Work out the finished part from the listing and answer in its coordinate system (mm). Face numbers are marked on the shaded views. A direction names the side the tool comes from. Give positions to 0.01 mm unless a question says otherwise; leave off trailing zeros. Loops run counter-clockwise (first coordinate to the right, second up) from the corner with the lowest first, then second, coordinate; pieces in that order, holes last. Notation, with made-up numbers: (-36.5, 73) -> (-3.5, 73) arc R17 cw to (-3.5, 96) -> close; hole circle Ø8 at (0.25, 19.5). An arc over 180 degrees is marked (long way). Answer as CSV lines item,"result". Start each with the question number.
1. Flat-ended cylindrical pins translate along their axes: pin 1 Ø0.6 at (y, z) = (1.5, 1) entering from -X; pin 2 Ø1.8 at (x, y) = (13, 2.5) entering from -Z; pin 3 Ø2 at (y, z) = (2, 6.5) entering from -X. Find the tip coordinate at first contact, or state that the pin passes through.
2. Find section A-A, the plane x = 0. Give the vertices of the cut face in (y, z).
3. Find section C-C, the plane z = 5.5. Give the vertices of the cut face in (x, y).
4. A tool of negligible diameter and unlimited length cuts with its end or side. For the marked faces 1, 2, 3 and 4, from which of +Z, -Z, +X, -X, +Y, -Y can it reach the whole face along a straight path? Write none if from no direction.
5. Find the intervals of material crossed by line 1 along X through (y, z) = (1.7, 2.25); line 2 along X through (y, z) = (2.8, -0.5); line 3 along Z through (x, y) = (0, 2.05), in increasing order.
6. Determine the mould class of the marked faces 5, 6, 7 and 8 for opening direction X: +X half, -X half, draft (parallel to the pull), parting line (faces both ways), or undercut.
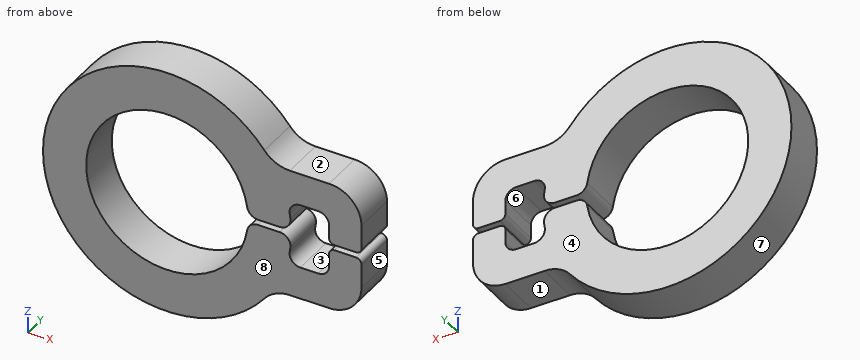
from build123d import *

# Parameters (mm, degrees)
BOSS_EXTRUDE1_DEPTH = 4
FILLET1_R           = 1
FILLET2_R           = 1
FILLET3_R           = 0.5
FILLET4_R           = 3


with BuildPart() as part:
    # Sketch1 → Boss-Extrude1 (new body)
    with BuildSketch(Plane(origin=(0, 0, 0), x_dir=(1, 0, 0), z_dir=(0, 1, 0))):
        with BuildLine():
            Line((9.810708435, 6), (18, 6))
            Line((18, 6), (18, 0.25))
            Line((18, 0.25), (15, 0.25))
            Line((15, 0.25), (15, 3))
            Line((15, 3), (11.101801656, 3))
            ThreePointArc((11.101801656, 3), (11.38289391, 1.636986937), (11.497282288, 0.25))
            Line((11.497282288, 0.25), (7.495832175, 0.25))
            ThreePointArc((7.495832175, 0.25), (-7.5, 0), (7.495832175, -0.25))
            Line((7.495832175, -0.25), (11.497282288, -0.25))
            ThreePointArc((11.497282288, -0.25), (11.38289391, -1.636986937), (11.101801656, -3))
            Line((11.101801656, -3), (15, -3))
            Line((15, -3), (15, -0.25))
            Line((15, -0.25), (18, -0.25))
            Line((18, -0.25), (18, -6))
            Line((18, -6), (9.810708435, -6))
            ThreePointArc((9.810708435, -6), (-11.5, 0), (9.810708435, 6))
        make_face()
    extrude(amount=BOSS_EXTRUDE1_DEPTH)

    # Fillet1
    fillet1_edges = [part.edges().sort_by_distance(p)[0] for p in [
        (11.497282288, 2, -0.25),
        (7.495832175, 2, -0.25),
        (7.495832175, 2, 0.25),
        (11.497282288, 2, 0.25),
    ]]
    fillet(fillet1_edges, radius=FILLET1_R)

    # Fillet2
    fillet2_edges = [part.edges().sort_by_distance(p)[0] for p in [
        (15, 2, -3),
        (11.101801656, 2, -3),
        (11.101801656, 2, 3),
        (15, 2, 3),
    ]]
    fillet(fillet2_edges, radius=FILLET2_R)

    # Fillet3
    fillet3_edges = [part.edges().sort_by_distance(p)[0] for p in [
        (18, 2, -0.25),
        (15, 2, -0.25),
        (15, 2, 0.25),
        (18, 2, 0.25),
    ]]
    fillet(fillet3_edges, radius=FILLET3_R)

    # Fillet4
    fillet4_edges = [part.edges().sort_by_distance(p)[0] for p in [
        (9.810708435, 2, -6),
        (18, 2, -6),
        (18, 2, 6),
        (9.810708435, 2, 6),
    ]]
    fillet(fillet4_edges, radius=FILLET4_R)


solid = part.part
Resolved:
1,pin 1,"stops at x = -11.48"
1,pin 2,"stops at z = -6"
1,pin 3,"stops at x = -10.1"
2,outline,"(0, -11.5) -> (4, -11.5) -> (4, -7.5) -> (0, -7.5) -> close; (0, 7.5) -> (4, 7.5) -> (4, 11.5) -> (0, 11.5) -> close"
3,outline,"(-10.1, 0) -> (-5.1, 0) -> (-5.1, 4) -> (-10.1, 4) -> close; (5.1, 0) -> (16.66, 0) -> (16.66, 4) -> (5.1, 4) -> close"
4,face 1,"-Z, +X, +Y, -Y"
4,face 2,"+Z, +X, +Y, -Y"
4,face 3,"+Y, -Y"
4,face 4,"+Z, -Z, +X, -X, +Y"
5,line 1,"x = -11.28 to -7.15, 7.15 to 11.37, 14.97 to 18"
5,line 2,"x = -11.49 to -7.48, 7.75 to 11.09, 15.07 to 17.93"
5,line 3,"z = -11.5 to -7.5, 7.5 to 11.5"
6,face 5,"+X half"
6,face 6,"undercut"
6,face 7,"parting line"
6,face 8,"draft"
